Geometry: final body of the model. Coordinates: model frame, mm. A direction names the side the tool comes from. Coordinates: 2 decimals unless noted, no trailing zeros. Loops run counter-clockwise (first coordinate to the right, second up) from the corner with the lowest first, then second, coordinate; pieces in that order, holes last. Notation, with made-up numbers: (-39.75, 69) -> (-13.75, 69) arc R21 ccw to (-13.75, 104) -> close; hole circle Ø6 at (12.25, 28.25). An arc over 180 degrees is marked (long way). One line per item, written item: value. Start each with the question number.
Item 1: Ray query, probe 1 along Z at (x, y) = (-16.5, 1); probe 2 along X at (y, z) = (-3, 17.5); probe 3 along X at (y, z) = (-4, 43). Return the intervals inside material, ascending. Write a range as from..to.
Item 2: Section query B-B on x = -11.5. Return loops of the section in (y, z), then the cut area to 3 significant figures.
Item 3: Section query C-C on z = 51. Return loops of the section in (x, y).
Item 4: Section query D-D on x = -19.5. Return loops of the section in (y, z).
Item 5: Contact query for flat-ended pins moving along their axis: pin 1 Ø5 at (x, z) = (-18, 13) entering from +Y; pin 2 Ø10 at (x, z) = (-0.5, 36) entering from -Y; pin 3 Ø4 at (x, z) = (-9, 34) entering from +Y; pin 4 Ø6 at (x, z) = (-1.5, 21.5) entering from +Y. Output: stop coordinate, or through.
Item 6: Set-up query: faces 1 (the flat face through (-11, -11, 10)), 2 (the flat face through (21, 0, 35)), 3 (the flat face through (0, 0, 0)). Return all of +Z, -Z, +X, -X, +Y, -Y with unobstructed straight access to the full face (end or side cutting, diameter ignored); none if empty.
Item 7: Section query A-A on y = 0. Return loops of the section in (x, z).
Autodesk Inventor part; units mm, degrees
ref_plane "YZ Plane" through (0, 0, 0) normal (1, 0, 0) x (0, 1, 0)
ref_plane "XZ Plane" through (0, 0, 0) normal (0, 1, 0) x (-1, 0, 0)
ref_plane "XY Plane" through (0, 0, 0) normal (0, 0, 1) x (1, 0, 0)
sketch "草圖1" plane through (0, 0, 0) normal (0, 0, 1) x (1, 0, 0)
  circle A0 centre (0, 0) radius 25
  dimension "d0" = 50
extrude "擠出1" add sketch "草圖1" along normal blind 10
sketch "草圖2" plane through (0, 0, 10) normal (0, 0, 1) x (1, 0, 0)
  circle A0 centre (6, 0) radius 19
  circle A1 centre (0, 0) radius 25
  dimension "d3" = 6
extrude "擠出2" add sketch "草圖2" along normal blind 50 contours A0
sketch "草圖3" plane through (6, 0, 60) normal (0, 0, 1) x (1, 0, 0)
  circle A0 centre (0, 0) radius 19
  circle A1 centre (0, 0) radius 19
  line L0 (15, 11.6619) -> (15, -11.6619)
  point P0 (-6, 0)
  point P1 (19, 0)
  point P2 (15, 11.6619)
  point P3 (15, -11.6619)
  dimension "d6" = 15
extrude "擠出3" cut sketch "草圖3" against normal up to surface (50 mm away) contours A0 L0 picked at (16.3333, 0)
properties part number "input"
Reply:
1. probe 1: z = 0..10
1. probe 2: x = -12.76..21
1. probe 3: x = -12.57..21
2. outline: (-22.2, 0) -> (22.2, 0) -> (22.2, 10) -> (7.4, 10) -> (7.4, 60) -> (-7.4, 60) -> (-7.4, 10) -> (-22.2, 10) -> close
2. area: 1,180 mm²
3. outline: (21, -11.66) -> (21, 11.66) arc R19 ccw (long way) to start
4. outline: (-15.64, 0) -> (15.64, 0) -> (15.64, 10) -> (-15.64, 10) -> close
5. pin 1: passes through
5. pin 2: stops at y = -18.94
5. pin 3: stops at y = 13.86
5. pin 4: stops at y = 18.46
6. face 1: +Z
6. face 2: +Z, +X, +Y, -Y
6. face 3: -Z, +X, -X, +Y, -Y
7. outline: (-25, 0) -> (25, 0) -> (25, 10) -> (21, 10) -> (21, 60) -> (-13, 60) -> (-13, 10) -> (-25, 10) -> close
